The listing builds one solid part. Answer for the finished solid, in the listing's coordinates (mm). Coordinates: 2 decimals unless noted, no trailing zeros. Order: outer loops, then holes, each group sorted by start corner. A loop starts at its lowest first (then second) coordinate and runs counter-clockwise, first axis right, second up. Notation, with made-up numbers: (-14.75, 59) -> (-5.75, 59) arc R12 ccw to (-5.75, 79) -> close; hole circle Ø5 at (-37.5, 28.25). An arc over 180 degrees is marked (long way). Answer in a Markdown table with one row per item.
```python
from build123d import *

# Parameters (mm, degrees)
F7_W      = 30
F7_H      = 30
F8_DEPTH  = 2100
F15_DEPTH = 15
F17_DEPTH = 15
F19_DEPTH = 15
F21_DEPTH = 15
F23_DEPTH = 15


with BuildPart() as f8:
    # F7 (on Top) → F8 (new body)
    with BuildSketch(Plane.XY):
        with Locations((-600, -15)):
            Rectangle(F7_W, F7_H)
    extrude(amount=F8_DEPTH)



with BuildPart() as f8b:
    # F7 (on Top) → F8, piece 2 (new body)
    with BuildSketch(Plane.XY):
        with Locations((600, -15)):
            Rectangle(F7_W, F7_H)
    extrude(amount=F8_DEPTH)


with BuildPart() as f8_1:
    add(f8.part)

    add(f8b.part)  # F15 merges F8b
    # F14 (on offset) → F15 (join)
    with BuildSketch(Plane.XY.offset(650)):
        with BuildLine():
            Line((585, 0), (0, 0))
            Line((0, 0), (-585, 0))
            Line((-585, 0), (-585, -30))
            Line((-585, -30), (-615, -30))
            Line((-615, -30), (-615, 0))
            Line((-615, 0), (-750, 0))
            Line((-750, 0), (-750, -360))
            ThreePointArc((-750, -360), (-738.2842712475, -388.2842712475), (-710, -400))
            Line((-710, -400), (0, -400))
            Line((0, -400), (710, -400))
            ThreePointArc((710, -400), (738.2842712475, -388.2842712475), (750, -360))
            Line((750, -360), (750, 0))
            Line((750, 0), (615, 0))
            Line((615, 0), (615, -30))
            Line((615, -30), (585, -30))
            Line((585, -30), (585, 0))
        make_face()
    extrude(amount=-F15_DEPTH)

    # F16 (on offset) → F17 (join)
    with BuildSketch(Plane.XY.offset(1000)):
        with BuildLine():
            Line((0, -400), (710, -400))
            ThreePointArc((710, -400), (738.2842712475, -388.2842712475), (750, -360))
            Line((750, -360), (750, 0))
            Line((750, 0), (615, 0))
            Line((615, 0), (615, -30))
            Line((615, -30), (585, -30))
            Line((585, -30), (585, 0))
            Line((585, 0), (0, 0))
            Line((0, 0), (-585, 0))
            Line((-585, 0), (-585, -30))
            Line((-585, -30), (-615, -30))
            Line((-615, -30), (-615, 0))
            Line((-615, 0), (-750, 0))
            Line((-750, 0), (-750, -360))
            ThreePointArc((-750, -360), (-738.2842712475, -388.2842712475), (-710, -400))
            Line((-710, -400), (0, -400))
        make_face()
    extrude(amount=-F17_DEPTH)

    # F18 (on offset) → F19 (join)
    with BuildSketch(Plane.XY.offset(1350)):
        with BuildLine():
            Line((0, -400), (710, -400))
            ThreePointArc((710, -400), (738.2842712475, -388.2842712475), (750, -360))
            Line((750, -360), (750, 0))
            Line((750, 0), (615, 0))
            Line((615, 0), (615, -30))
            Line((615, -30), (585, -30))
            Line((585, -30), (585, 0))
            Line((585, 0), (0, 0))
            Line((0, 0), (-585, 0))
            Line((-585, 0), (-585, -30))
            Line((-585, -30), (-615, -30))
            Line((-615, -30), (-615, 0))
            Line((-615, 0), (-750, 0))
            Line((-750, 0), (-750, -360))
            ThreePointArc((-750, -360), (-738.2842712475, -388.2842712475), (-710, -400))
            Line((-710, -400), (0, -400))
        make_face()
    extrude(amount=-F19_DEPTH)

    # F20 (on offset) → F21 (join)
    with BuildSketch(Plane.XY.offset(1700)):
        with BuildLine():
            Line((0, -400), (710, -400))
            ThreePointArc((710, -400), (738.2842712475, -388.2842712475), (750, -360))
            Line((750, -360), (750, 0))
            Line((750, 0), (615, 0))
            Line((615, 0), (615, -30))
            Line((615, -30), (585, -30))
            Line((585, -30), (585, 0))
            Line((585, 0), (0, 0))
            Line((0, 0), (-585, 0))
            Line((-585, 0), (-585, -30))
            Line((-585, -30), (-615, -30))
            Line((-615, -30), (-615, 0))
            Line((-615, 0), (-750, 0))
            Line((-750, 0), (-750, -360))
            ThreePointArc((-750, -360), (-738.2842712475, -388.2842712475), (-710, -400))
            Line((-710, -400), (0, -400))
        make_face()
    extrude(amount=-F21_DEPTH)

    # F22 (on offset) → F23 (join)
    with BuildSketch(Plane.XY.offset(2040)):
        with BuildLine():
            Line((0, -400), (710, -400))
            ThreePointArc((710, -400), (738.2842712475, -388.2842712475), (750, -360))
            Line((750, -360), (750, 0))
            Line((750, 0), (615, 0))
            Line((615, 0), (615, -30))
            Line((615, -30), (585, -30))
            Line((585, -30), (585, 0))
            Line((585, 0), (0, 0))
            Line((0, 0), (-585, 0))
            Line((-585, 0), (-585, -30))
            Line((-585, -30), (-615, -30))
            Line((-615, -30), (-615, 0))
            Line((-615, 0), (-750, 0))
            Line((-750, 0), (-750, -360))
            ThreePointArc((-750, -360), (-738.2842712475, -388.2842712475), (-710, -400))
            Line((-710, -400), (0, -400))
        make_face()
    extrude(amount=-F23_DEPTH)


solid = f8_1.part
```
(1) A cutting plane is placed at B-B, the plane x = -41.5. Determine the outline of the cut face in (y, z), then the cut area to 3 significant figures.
Check values:
| item | result |
|---|---|
| outline | (-400, 635) -> (0, 635) -> (0, 650) -> (-400, 650) -> close; (-400, 985) -> (0, 985) -> (0, 1000) -> (-400, 1000) -> close; (-400, 1335) -> (0, 1335) -> (0, 1350) -> (-400, 1350) -> close; (-400, 1685) -> (0, 1685) -> (0, 1700) -> (-400, 1700) -> close; (-400, 2025) -> (0, 2025) -> (0, 2040) -> (-400, 2040) -> close |
| area | 30,000 mm² |
(2) A cutting plane is placed at A-A, the plane y = -103. Determine the outline of the cut face in (x, z), then the cut area to 4 significant figures.
Check values:
| item | result |
|---|---|
| outline | (-750, 635) -> (750, 635) -> (750, 650) -> (-750, 650) -> close; (-750, 985) -> (750, 985) -> (750, 1000) -> (-750, 1000) -> close; (-750, 1335) -> (750, 1335) -> (750, 1350) -> (-750, 1350) -> close; (-750, 1685) -> (750, 1685) -> (750, 1700) -> (-750, 1700) -> close; (-750, 2025) -> (750, 2025) -> (750, 2040) -> (-750, 2040) -> close |
| area | 112,500 mm² |
(3) Flat-ended cylindrical pins translate along their axes: pin 1 (1 mm diameter, centred on x = -250, y = -125, fed in from -Z); pin 2 (15 mm diameter, centred on x = -596.5, z = 1240, fed in from -Y); pin 3 (1 mm diameter, centred on x = -516, y = -149.5, fed in from +Z); pin 4 (6 mm diameter, centred on x = 162, z = 988, fed in from +Y). Find the tip coordinate at first contact, or state that the pin passes through.
Check values:
| item | result |
|---|---|
| pin 1 | z = 635 |
| pin 2 | y = -30 |
| pin 3 | z = 2040 |
| pin 4 | y = 0 |
(4) A cutting plane is placed at C-C, the plane z = 1453.5. Determine the outline of the cut face in (x, y).
Check values:
| item | result |
|---|---|
| outline | (-615, -30) -> (-585, -30) -> (-585, 0) -> (-615, 0) -> close; (585, -30) -> (615, -30) -> (615, 0) -> (585, 0) -> close |
(5) For a pull along Z with two mould halves and no side action, classify faces 1 (the flat face through (-10, -197, 1335)), 2 (the cylindrical face through (737.972, -388.594, 1342.605)) as released by +Z, released by -Z, zero draft, split by the parting line, or undercut.
Check values:
| item | result |
|---|---|
| face 1 | undercut |
| face 2 | zero draft |
(6) Find the intervals of material crossed by line 1 along Z through (x, y) = (-26, -149); line 2 along Y through (x, z) = (594.5, 771.5), in increasing order. Write a range as from..to.
Check values:
| item | result |
|---|---|
| line 1 | 635..650, 985..1000, 1335..1350, 1685..1700, 2025..2040 |
| line 2 | -30..0 |
